Autodesk Inventor part; units mm, degrees
ref_plane "YZ Plane" through (0, 0, 0) normal (1, 0, 0) x (0, 1, 0)
ref_plane "XZ Plane" through (0, 0, 0) normal (0, 1, 0) x (-1, 0, 0)
ref_plane "XY Plane" through (0, 0, 0) normal (0, 0, 1) x (1, 0, 0)
sketch "草圖1" plane through (0, 0, 0) normal (1, 0, 0) x (0, 1, 0)
  line L0 (0, 0) -> (113.9, 0)
  circle A0 centre (113.9, 0) radius 6
  circle A1 centre (0, 0) radius 6
  circle A2 centre (0, 0) radius 9
  circle A3 centre (113.9, 0) radius 9
  line L1 (7.4833, 5) -> (17.4833, 5)
  line L2 (17.4833, 5) -> (19.4833, 3)
  line L3 (19.4833, 3) -> (94.4167, 3)
  line L4 (94.4167, 3) -> (96.4167, 5)
  line L5 (96.4167, 5) -> (106.4167, 5)
  line L6 (106.4167, -5) -> (96.4167, -5)
  line L7 (96.4167, -5) -> (94.4167, -3)
  line L8 (94.4167, -3) -> (19.4833, -3)
  line L9 (19.4833, -3) -> (17.4833, -5)
  line L10 (17.4833, -5) -> (7.4833, -5)
  dimension "d0" = 113.9
  dimension "d1" = 12
  dimension "d2" = 12
  dimension "d3" = 18
  dimension "d4" = 18
  dimension "d5" = 3
  dimension "d6" = 5
  dimension "d7" = 10
  dimension "d8" = 10
extrude "擠出1" add sketch "草圖1" along normal mid plane 5
fillet "圓角1" radius 4 12 edges at (0, 106.4167, 5) (0, 96.4167, 5) (0, 94.4167, 3) (0, 17.4833, 5) (0, 7.4833, 5) (0, 19.4833, 3) (0, 7.4833, -5) (0, 17.4833, -5) (0, 19.4833, -3) (0, 106.4167, -5) (0, 96.4167, -5) (0, 94.4167, -3)
equation "\"d2\" = d1"
equation "\"d3\" = d4"
equation "\"d8\" = d7"
properties part number "Link_DE" material "ABS 塑膠"
The listing builds one solid part. Answer for the finished solid, in the listing's coordinates (mm). A direction names the side the tool comes from. Coordinates: 2 decimals unless noted, no trailing zeros. Write each loop counter-clockwise with the first axis right and the second up, starting at its lowest first coordinate (ties: lowest second). Pieces come first, ordered by that corner, then holes. Notation, with made-up numbers: (-18, 87.25) - (-9, 87.25) arc R12 ccw to (-9, 102.25) - close; hole circle Ø10 at (26, 10.5). An arc over 180 degrees is marked (long way). One line per item, written item: value.
1) Find section C-C (z = 7.5). Give the vertices of the cut face in (x, y).
Geometry check:
outline: (-2.5, -4.97) - (2.5, -4.97) - (2.5, 4.97) - (-2.5, 4.97) - close; (-2.5, 108.93) - (2.5, 108.93) - (2.5, 118.87) - (-2.5, 118.87) - close
2) For a pull along Y with two mould halves and no side action, classify faces 1 (the flat face through (0, 13, -5)), 2 (the cylindrical face through (0, -9, 0)), 3 (the flat face through (-2.5, 56, 0)) as pulls with the +Y half, pulls with the -Y half, needs draft (parallel to the pull), parting line crosses it, or undercut.
Geometry check:
face 1: undercut
face 2: undercut
face 3: needs draft
3) Each of these flat-tipped pins is pushed along its axis until it touches: pin 1 Ø3 at (x, y) = (-1.5, 65) entering from -Z; pin 2 Ø1.5 at (x, y) = (-1, 100) entering from +Z. Where does it stop, or does it pass through?
Geometry check:
pin 1: stops at z = -3
pin 2: stops at z = 5
4) Consider line 1 along Z through (x, y) = (-1.3, 113.9); line 2 along Y through (x, z) = (-1.9, -2.75); line 3 along Y through (x, z) = (-0.4, -4). Determine where each line is inside the solid, lowest interval first. Write a range as from..to.
Geometry check:
line 1: z = -9..-6, 6..9
line 2: y = -8.57..-5.33, 5.33..108.57, 119.23..122.47
line 3: y = -8.06..-4.47, 4.47..18.49, 95.41..109.43, 118.37..121.96
5) Find section A-A (y = 113.9). Give the vertices of the cut face in (x, z).
Geometry check:
outline: (-2.5, -9) - (2.5, -9) - (2.5, -6) - (-2.5, -6) - close; (-2.5, 6) - (2.5, 6) - (2.5, 9) - (-2.5, 9) - close
6) Find section B-B (z = 0). Give the vertices of the cut face in (x, y), and give its area (4 significant figures).
Geometry check:
outline: (-2.5, -9) - (2.5, -9) - (2.5, -6) - (-2.5, -6) - close; (-2.5, 6) - (2.5, 6) - (2.5, 107.9) - (-2.5, 107.9) - close; (-2.5, 119.9) - (2.5, 119.9) - (2.5, 122.9) - (-2.5, 122.9) - close
area: 539.5 mm2
7) A tool of negligible diameter and unlimited length cuts with its end or side. For faces 4 (the cylindrical face through (0.04, 7.79, 5.33)), 5 (the cylindrical face through (0.04, 106.11, -5.33)), 6 (the cylindrical face through (0, -6, 0)), from which of +Z, -Z, +X, -X, +Y, -Y can it reach the whole face along a straight path? Write none if from no direction.
Geometry check:
face 4: +Z, +X, -X
face 5: -Z, +X, -X
face 6: +X, -X
8) Find section D-D (x = 1.65). Count the separate pieces of the cut face and the enclosed holes in it, and give its area (3 significant figures).
Geometry check:
separate pieces: 1
enclosed holes: 2
area: 946 mm2
